CAD build for the part. Positions are in the model's coordinates, mm. Coordinates: 2 decimals unless noted, no trailing zeros. Write each loop counter-clockwise with the first axis right and the second up, starting at its lowest first coordinate (ties: lowest second). Pieces come first, ordered by that corner, then holes. Notation, with made-up numbers: M 40.25,73.5 L 67.25,73.5 A28 ccw 67.25,97.5 Z; hole C 79,26.25 d11. An arc over 180 degrees is marked long. Put each result on its own line as item: value. Start each with the question number.
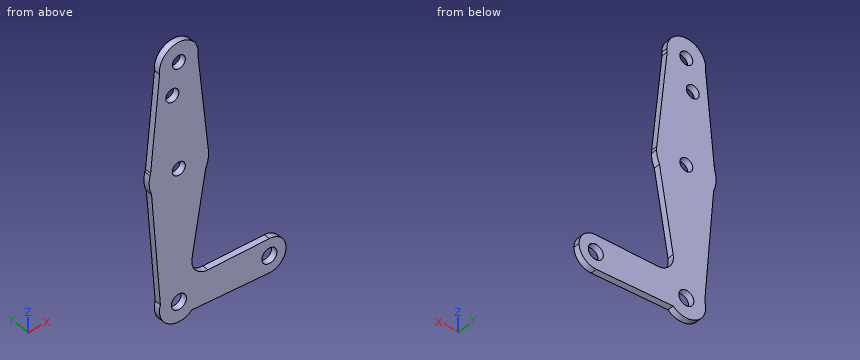
```python
from build123d import *

# Parameters (mm, degrees)
F0_R     = 3.175
F0_R_2   = 3.6935498759
F1_DEPTH = 3.048


# Not quite as in the source:
# - the program builds the solid bodies; features that only make, move or delete a surface that nothing else refers to are left out


with BuildPart() as f1:
    # F0 (on Front) → F1 (new body)
    with BuildSketch(Plane.XZ):
        with BuildLine():
            ThreePointArc((9.3833145649, 112.6632248852), (9.4895125331, 113.4785519586), (9.525, 114.3))
            ThreePointArc((9.525, 114.3), (-0.6480489734, 123.8029288921), (-9.4368178537, 113.0069053411))
            ThreePointArc((-9.4368178537, 113.0069053411), (-0.1739100757, 104.7765877814), (9.3833145649, 112.6632248852))
        make_face()
        with Locations((0, 114.3)):
            Circle(F0_R, mode=Mode.SUBTRACT)
        with BuildLine():
            ThreePointArc((9.3833145649, 112.6632248852), (-0.1739100757, 104.7765877814), (-9.4368178537, 113.0069053411))
            Line((-9.4368178537, 113.0069053411), (-13.8405466215, 68.1295922048))
            ThreePointArc((-13.8405466215, 68.1295922048), (1.5694846966, 78.00967169), (14.510379821, 65.0629242514))
            Line((14.510379821, 65.0629242514), (9.3833145649, 112.6632248852))
        make_face()
        with Locations((-3.175, 99.886942851)):
            Circle(F0_R, mode=Mode.SUBTRACT)
        with BuildLine():
            ThreePointArc((14.510379821, 65.0629242514), (1.5694846966, 78.00967169), (-13.8405466215, 68.1295922048))
            ThreePointArc((-13.8405466215, 68.1295922048), (-14.0055954943, 67.6033095928), (-14.1506404779, 67.0711663123))
            Line((-14.1506404779, 67.0711663123), (-13.406906479, 57.7338302637))
            ThreePointArc((-13.406906479, 57.7338302637), (-0.26538464, 48.9081041068), (13.1883694151, 57.2501386467))
            Line((13.1883694151, 57.2501386467), (14.510379821, 65.0629242514))
        make_face()
        with Locations((0, 63.5)):
            Circle(F0_R, mode=Mode.SUBTRACT)
        with BuildLine():
            ThreePointArc((14.5943089855, 63.5), (14.5733115895, 64.2825880654), (14.510379821, 65.0629242514))
            Line((14.510379821, 65.0629242514), (13.1883694151, 57.2501386467))
            ThreePointArc((13.1883694151, 57.2501386467), (14.2384864544, 60.2969767012), (14.5943089855, 63.5))
        make_face()
        with BuildLine():
            Line((-13.406906479, 57.7338302637), (-14.1506404779, 67.0711663123))
            ThreePointArc((-14.1506404779, 67.0711663123), (-14.5482321844, 62.3412096509), (-13.406906479, 57.7338302637))
        make_face()
        with BuildLine():
            Line((6.4543763873, 17.4537470642), (13.1883694151, 57.2501386467))
            ThreePointArc((13.1883694151, 57.2501386467), (-0.26538464, 48.9081041068), (-13.406906479, 57.7338302637))
            Line((-13.406906479, 57.7338302637), (-9.0459006939, 2.9828351674))
            ThreePointArc((-9.0459006939, 2.9828351674), (1.5105331659, 9.4044624809), (9.525, 0))
            ThreePointArc((9.525, 0), (8.7148100466, -3.8441788267), (6.4220685875, -7.0343912357))
            Line((6.4220685875, -7.0343912357), (44.2035880522, -8.173426155))
            ThreePointArc((44.2035880522, -8.173426155), (36.2737887259, 0.1232199644), (44.45, 8.1771397175))
            Line((44.45, 8.1771397175), (14.2931469281, 8.1771397175))
            ThreePointArc((14.2931469281, 8.1771397175), (8.220631645, 10.996039865), (6.4543763873, 17.4537470642))
        make_face()
        with BuildLine():
            ThreePointArc((9.525, 0), (1.5105331659, 9.4044624809), (-9.0459006939, 2.9828351674))
            ThreePointArc((-9.0459006939, 2.9828351674), (-5.1775795439, -7.9948918108), (6.4220685875, -7.0343912357))
            ThreePointArc((6.4220685875, -7.0343912357), (8.7148100466, -3.8441788267), (9.525, 0))
        make_face()
        Circle(F0_R_2, mode=Mode.SUBTRACT)
        with BuildLine():
            ThreePointArc((52.6271397175, 0), (50.2321109449, 5.7821109449), (44.45, 8.1771397175))
            ThreePointArc((44.45, 8.1771397175), (36.2737887259, 0.1232199644), (44.2035880522, -8.173426155))
            ThreePointArc((44.2035880522, -8.173426155), (50.1443247639, -5.8685841088), (52.6271397175, 0))
        make_face()
        with Locations((44.45, 0)):
            Circle(F0_R_2, mode=Mode.SUBTRACT)
    extrude(amount=F1_DEPTH)


solid = f1.part
```
(1) Drop flat-ended pins along their axis: pin 1 (9.5 mm diameter, centred on x = 0, z = 0, fed in from -Y); pin 2 (1.5 mm diameter, centred on y = -1, z = 33, fed in from -X). Give the stop position or say it passes through.
(2) Drill centre lines: line 1 (X direction, y = -1.85, z = -1.5); line 2 (Z direction, x = 44.45, y = -1.4); line 3 (X direction, y = -0.5, z = 113.5). Where is each one in solid material? Low to high. Write a range as [from, to].
(3) Slice it at A-A, the plane y = -0.7. Write the cut outline in (x, z) (3 decimals), then the cut area to 3 significant figures.
(4) Slice it at B-B, the plane x = 22.5. Write the cut outline in (y, z), then the cut area to 3 significant figures.
(5) Slice it at C-C, the plane z = 33.5. Write the cut outline in (x, y), then the cut area to 3 significant figures.
Result set:
1. pin 1: stops at y = -3.05
1. pin 2: stops at x = -11.5
2. line 1: x = [-9.41, -3.38], [3.38, 41.07], [47.83, 52.49]
2. line 2: z = [-8.18, -3.69], [3.69, 8.18]
2. line 3: x = [-9.49, -3.07], [3.07, 9.49]
3. outline: M -13.841,68.13 A14.594 ccw -13.407,57.734 L -9.046,2.983 A9.525 ccw 6.422,-7.034 L 44.204,-8.173 A8.177 ccw long 44.45,8.177 L 14.293,8.177 A7.95 cw 6.454,17.454 L 13.188,57.25 A14.594 ccw 14.51,65.063 L 9.383,112.663 A9.525 ccw long -9.437,113.007 Z; hole C -3.175,99.887 d6.35; hole C 0,0 d7.387; hole C 0,63.5 d6.35; hole C 0,114.3 d6.35; hole C 44.45,0 d7.387
3. area: 3,330 mm^2
4. outline: M -3.05,-7.52 L 0,-7.52 L 0,8.18 L -3.05,8.18 Z
4. area: 47.8 mm^2
5. outline: M -11.48,-3.05 L 9.17,-3.05 L 9.17,0 L -11.48,0 Z
5. area: 62.9 mm^2
